```python
from build123d import *

# Parameters (mm, degrees)
SKETCH2_W               = 125
SKETCH2_H               = 125
BOSS_EXTRUDE1_DEPTH     = 20
CUT_EXTRUDE1_DEPTH      = 178.904468747
CUT_EXTRUDE1_DEPTH_BACK = 178.904468747
BOSS_EXTRUDE2_DEPTH     = 10
CUT_EXTRUDE2_DEPTH      = 1
CUT_EXTRUDE3_DEPTH      = 1


with BuildPart() as part:
    # Sketch2 → Boss-Extrude1 (new body)
    with BuildSketch(Plane(origin=(0, 0, 0), x_dir=(1, 0, 0), z_dir=(0, 1, 0))):
        with Locations((62.5, 62.5)):
            Rectangle(SKETCH2_W, SKETCH2_H)
    extrude(amount=BOSS_EXTRUDE1_DEPTH)

    # Sketch4 → Cut-Extrude1 (cut, two sides: drawn at the far end of the back side and taken through both)
    with BuildSketch(Plane(origin=(125, 0, 0), x_dir=(0, 0, -1), z_dir=(1, 0, 0)).offset(-CUT_EXTRUDE1_DEPTH_BACK)):
        Polygon((-98.875201044, 237.750402088), (10, 20), (15, 10), (110, 10), (115, 20), (223.875201044, 237.750402088), (223.875201044, 724.655103285), (-98.875201044, 724.655103285), align=None)
    extrude(amount=CUT_EXTRUDE1_DEPTH + CUT_EXTRUDE1_DEPTH_BACK, mode=Mode.SUBTRACT)

    # Sketch3 → Boss-Extrude2 (add)
    with BuildSketch(Plane.XY):
        with BuildLine():
            Line((57.5, 20), (57.5, 90))
            add(Edge.make_bspline(
                [(57.5, 90), (62.5, 130), (67.5, 90)],
                knots=[0, 0, 0, 1, 1, 1], degree=2))
            Line((67.5, 90), (67.5, 20))
            Line((67.5, 20), (57.5, 20))
        make_face()
    boss_extrude2 = extrude(amount=-BOSS_EXTRUDE2_DEPTH)

    # Sketch6 → Cut-Extrude2 (cut)
    with BuildSketch(Plane.XY):
        with BuildLine():
            Line((57.5, 20), (67.5, 20))
            Line((67.5, 20), (67.5, 90))
            add(Edge.make_bspline(
                [(67.5, 90), (62.500000001, 129.999999993), (57.500000002, 90.000000015)],
                knots=[0, 0, 0, 1, 1, 1], degree=2))
            Line((57.500000002, 90.000000015), (57.5, 20))
        make_face()
    cut_extrude2 = extrude(amount=-CUT_EXTRUDE2_DEPTH, mode=Mode.SUBTRACT)

    # Sketch7 → Cut-Extrude3 (cut)
    with BuildSketch(Plane(origin=(0, 0, -10), x_dir=(-1, 0, 0), z_dir=(0, 0, -1))):
        with BuildLine():
            Line((-67.5, 20), (-57.5, 20))
            Line((-57.5, 20), (-57.5, 90))
            add(Edge.make_bspline(
                [(-57.5, 90), (-62.499999999, 129.999999993), (-67.499999998, 90.000000015)],
                knots=[0, 0, 0, 1, 1, 1], degree=2))
            Line((-67.499999998, 90.000000015), (-67.5, 20))
        make_face()
    cut_extrude3 = extrude(amount=-CUT_EXTRUDE3_DEPTH, mode=Mode.SUBTRACT)

    # Mirror1: Boss-Extrude2, Cut-Extrude2, Cut-Extrude3 across plane
    add(boss_extrude2.mirror(Plane.XY.offset(-62.5)))
    add(cut_extrude2.mirror(Plane.XY.offset(-62.5)), mode=Mode.SUBTRACT)
    add(cut_extrude3.mirror(Plane.XY.offset(-62.5)), mode=Mode.SUBTRACT)


solid = part.part
```
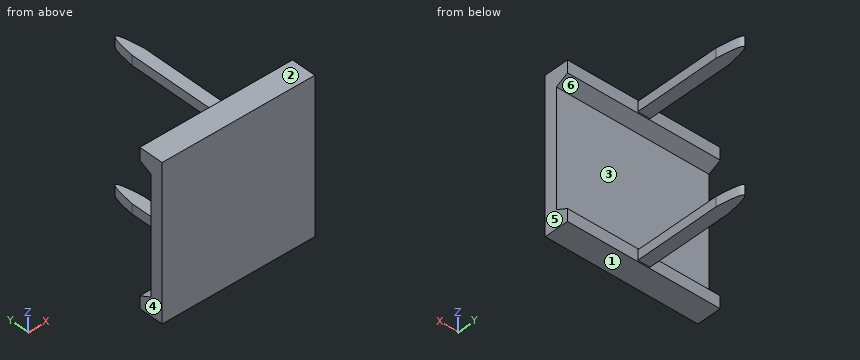
The listing builds one solid part. Answer for the finished solid, in the listing's coordinates (mm). Face numbers are marked on the shaded views. A direction names the side the tool comes from. Coordinates: 2 decimals unless noted, no trailing zeros. Loops run counter-clockwise (first coordinate to the right, second up) from the corner with the lowest first, then second, coordinate; pieces in that order, holes last. Notation, with made-up numbers: (23.5, -35.75) -> (52.5, -35.75) arc R18 cw to (52.5, -27.75) -> close; hole circle Ø1 at (37.5, -19.5). An arc over 180 degrees is marked (long way). Use one line per item in the form item = value. Start each with the question number.
Item 1: The mould has two halves that part along Z. Classify the marked faces 1, 2, 3 and 4: released by +Z, released by -Z, zero draft, split by the parting line, or undercut.
Item 2: The part is cut by section B-B on x = 37. Determine the outline of the cut face in (y, z).
Item 3: Flat-ended cylindrical pins translate along their axes: pin 1 Ø3 at (x, y) = (64, 50) entering from -Z; pin 2 Ø1.5 at (x, z) = (107.5, -19.5) entering from +Y; pin 3 Ø2.5 at (y, z) = (66, -5) entering from +X; pin 4 Ø2 at (x, z) = (104, -112.5) entering from -Y. Find the tip coordinate at first contact, or state that the pin passes through.
Item 4: A tool of negligible diameter and unlimited length cuts with its end or side. For the marked faces 5 and 6, from which of +Z, -Z, +X, -X, +Y, -Y can it reach the whole face along a straight path? Write none if from no direction.
Item 5: The part is cut by section C-C on z = -31. Determine the outline of the cut face in (x, y), then the cut area to 3 significant figures.
Item 6: Consider L1, parallel to Y at x = 12, z = -47.5; L2, parallel to Z at x = 100.5, y = 12; L3, parallel to Y at x = 62.5, z = -110.5. Determine where each line is inside the solid, lowest interval first. Write a range as [from, to].
Item 7: The part is cut by section A-A on y = 87. Determine the outline of the cut face in (x, z), then the cut area to 3 significant figures.
Item 8: The part is cut by section D-D on z = -113. Determine the outline of the cut face in (x, y).
Answer key:
q1.face_1 = released by -Z
q1.face_2 = released by +Z
q1.face_3 = undercut
q1.face_4 = zero draft
q2.outline = (0, -125) -> (20, -125) -> (20, -115) -> (10, -110) -> (10, -15) -> (20, -10) -> (20, 0) -> (0, 0) -> close
q3.pin_1 = -124
q3.pin_2 = 10
q3.pin_3 = 67.5
q3.pin_4 = 0
q4.face_5 = +Z, -Z, +X, +Y, -Y
q4.face_6 = +X, -X, +Y
q5.outline = (0, 0) -> (125, 0) -> (125, 10) -> (0, 10) -> close
q5.area = 1,250 mm2
q6.L1 = [0, 10]
q6.L2 = [-125, -111], [-14, 0]
q6.L3 = [0, 11]
q7.outline = (57.5, -124) -> (67.5, -124) -> (67.5, -116) -> (57.5, -116) -> close; (57.5, -9) -> (67.5, -9) -> (67.5, -1) -> (57.5, -1) -> close
q7.area = 160 mm2
q8.outline = (0, 0) -> (125, 0) -> (125, 16) -> (0, 16) -> close
